Here's how the part is built. I have some questions about the finished solid (model axes, mm). Face numbers are marked on the shaded views. A direction names the side the tool comes from. Coordinates: 2 decimals unless noted, no trailing zeros. Write each loop counter-clockwise with the first axis right and the second up, starting at its lowest first coordinate (ties: lowest second). Pieces come first, ordered by that corner, then holes. Notation, with made-up numbers: M -24,-6 L -20,-6 A15 cw -20,2 Z; hole C -20.5,30.25 d6. An arc over 180 degrees is marked long. Use one line per item in the form item = value. Start each with the question number.
1. On a 3-axis mill with a long thin cutter (end or side, diameter ignored), from which of +Z, -Z, +X, -X, +Y, -Y can I reach the whole of each face in a straight line? I mean the marked faces 4, 5 and 6. Say none if no direction works.
2. I want a section at D-D, the plane y = -6.5. List the corners of the cut face in (x, z) for me.
3. I want a section at B-B, the plane y = -1.5. List the corners of the cut face in (x, z) for me.
4. I'm going to push flat-ended pins straight in: pin 1 Ø8 at (x, z) = (-2.5, 54.5) entering from -Y; pin 2 Ø5 at (x, y) = (-7.5, -5.5) entering from +Z; pin 3 Ø1.5 at (y, z) = (-6.5, 46) entering from -X; pin 4 Ø5.5 at (y, z) = (-8.5, 42.5) entering from +X. Where does each tip first touch, or does it pass through?
5. Please list where these lines run through material, in increasing order: line 1 along X through (y, z) = (-3.45, 50); line 2 along Z through (x, y) = (10, -2.1); line 3 along Y through (x, z) = (-17.5, 45.5). Write a range as [from, to].
6. I want a section at C-C, the plane z = 47.25. List the corners of the cut face in (x, y) for me, plus the area to 3 significant figures.
7. I want a section at A-A, the plane x = 10. List the corners of the cut face in (y, z) for me, plus the area to 3 significant figures.
8. Thinking about a two-plate mould opening in X: for the marked faces 1, 2 and 3, which applies, released by +X, released by -X, zero draft, split by the parting line, or undercut?
from build123d import *

# Parameters (mm, degrees)
F0_W     = 17.5
F0_H     = 21.2181335688
F0_W_2   = 5
F1_DEPTH = 5
F2_W     = 5
F2_H     = 11.2181335688
F3_DEPTH = 5
F4_D     = 4.5
F4_DEPTH = 17
F4_TIP   = 1.3519363928


with BuildPart() as f1:
    # F0 (on Front) → F1 (new body)
    with BuildSketch(Plane.XZ):
        with Locations((-11.25, 49.3909332156)):
            Rectangle(F0_W, F0_H)
        with Locations((0, 49.3909332156)):
            Rectangle(F0_W_2, F0_H)
        with Locations((11.25, 49.3909332156)):
            Rectangle(F0_W, F0_H)
    extrude(amount=F1_DEPTH)

    # F2 (on face) → F3 (join)
    with BuildSketch(Plane.XZ.offset(5)):
        with Locations((0, 44.3909332156)):
            Rectangle(F2_W, F2_H)
    extrude(amount=F3_DEPTH)

    # F4
    with Locations(Plane(origin=(0, 0, 0), x_dir=(1, 0, 0), z_dir=(0, 1, 0))):
        with Locations((10, -50), (-10, -50)):
            Hole(F4_D / 2, depth=F4_DEPTH)
            with Locations((0, 0, -(F4_DEPTH + F4_TIP / 2))):  # 118° drill point
                Cone(0, F4_D / 2, F4_TIP, mode=Mode.SUBTRACT)


solid = f1.part
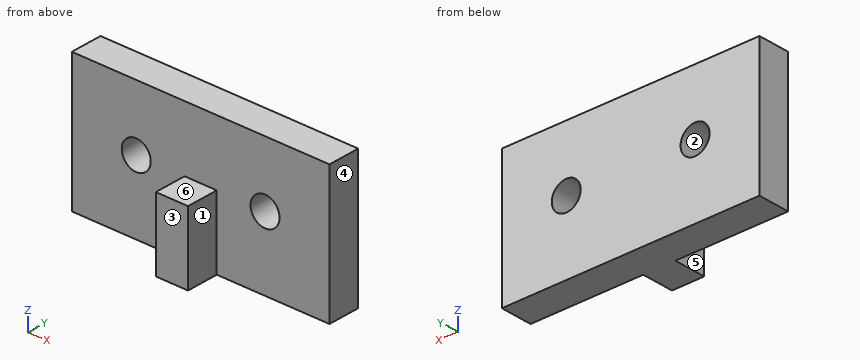
Answer list:
q1.face_4 = +Z, -Z, +X, +Y, -Y
q1.face_5 = +Z, -Z, -X, -Y
q1.face_6 = +Z, +X, -X, -Y
q2.outline = M -2.5,38.78 L 2.5,38.78 L 2.5,50 L -2.5,50 Z
q3.outline = M -20,38.78 L 20,38.78 L 20,60 L -20,60 Z; hole C -10,50 d4.5; hole C 10,50 d4.5
q4.pin_1 = -5
q4.pin_2 = 60
q4.pin_3 = -2.5
q4.pin_4 = 2.5
q5.line_1 = [-20, -12.25], [-7.75, 7.75], [12.25, 20]
q5.line_2 = [38.78, 47.75], [52.25, 60]
q5.line_3 = [-5, 0]
q6.outline = M -20,-5 L -2.5,-5 L -2.5,-10 L 2.5,-10 L 2.5,-5 L 20,-5 L 20,0 L -20,0 Z
q6.area = 225 mm²
q7.outline = M -5,38.78 L 0,38.78 L 0,47.75 L -5,47.75 Z; M -5,52.25 L 0,52.25 L 0,60 L -5,60 Z
q7.area = 83.6 mm²
q8.face_1 = released by +X
q8.face_2 = undercut
q8.face_3 = zero draft
